from build123d import *

# Parameters (mm, degrees)
SKETCH1_W            = 190.5
SKETCH1_H            = 76.2
BOSS_EXTRUDE1_DEPTH  = 3.175
SKETCH2_R            = 1.545336663
CUT_EXTRUDE4_DEPTH   = 4.175
SKETCH3_W            = 153.75
SKETCH3_H            = 3.175
BOSS_EXTRUDE2_DEPTH  = 3.175
CUT_SWEEP1_PROFILE_R = 12.7


with BuildPart() as part:
    # Sketch1 → Boss-Extrude1 (new body)
    with BuildSketch(Plane(origin=(0, 0, 0), x_dir=(1, 0, 0), z_dir=(0, 1, 0))):
        Rectangle(SKETCH1_W, SKETCH1_H)
    extrude(amount=BOSS_EXTRUDE1_DEPTH)

    # Sketch2 → Cut-Extrude4 (cut, through all)
    with BuildSketch(Plane(origin=(0, 3.175, 0), x_dir=(1, 0, 0), z_dir=(0, 1, 0))):
        Polygon((-58.5, 12.6), (-58.5, -38.1), (95.25, -38.1), (95.25, 38.1), (58.5, 38.1), (58.5, 12.6), (56.5, 12.6), (41.5, 26.6), (41.5, 32.45), (-41.5, 32.45), (-41.5, 26.6), (-56.5, 12.6), align=None)
        with Locations((-52.505245516, 25.605245516)):
            Circle(SKETCH2_R)
        with Locations((52.5, 25.605245516)):
            Circle(SKETCH2_R)
    extrude(amount=-CUT_EXTRUDE4_DEPTH, mode=Mode.SUBTRACT)

    # Sketch3 → Boss-Extrude2 (add)
    with BuildSketch(Plane(origin=(0, 0, -38.1), x_dir=(-1, 0, 0), z_dir=(0, 0, -1))):
        with Locations((18.375, 1.5875)):
            Rectangle(SKETCH3_W, SKETCH3_H)
    extrude(amount=BOSS_EXTRUDE2_DEPTH)

    # Cut-Sweep1: sweep along a curve in space
    with BuildLine() as cut_sweep1_path:
        Line((-96.6, 3.175, 467.883912637), (-96.6, 3.175, -36.654630794))
        Line((-96.6, 3.175, -36.654630794), (-96.6, 3.175, -207.159673584))
    # Cut-Sweep1 profile (on start of the path) → Cut-Sweep1 (sweep, cut)
    with BuildSketch(Plane(origin=(-96.6, 3.175, 467.883912637), x_dir=(0, -1, 0), z_dir=(0, 0, -1))):
        Circle(CUT_SWEEP1_PROFILE_R)
    sweep(path=cut_sweep1_path.line, mode=Mode.SUBTRACT)


solid = part.part
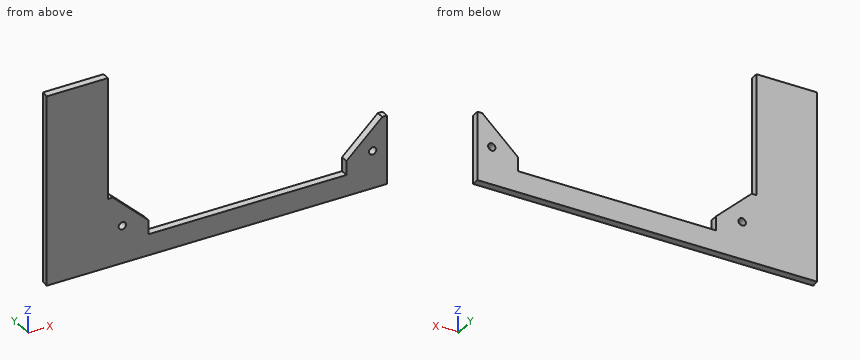
CAD build for the part. Positions are in the model's coordinates, mm. Coordinates: 2 decimals unless noted, no trailing zeros. Order: outer loops, then holes, each group sorted by start corner. A loop starts at its lowest first (then second) coordinate and runs counter-clockwise, first axis right, second up. Notation, with made-up numbers: (-17.75, 35) -> (-13.75, 35) arc R20 cw to (-13.75, 41) -> close; hole circle Ø5 at (-30, 34.5). An arc over 180 degrees is marked (long way). Answer in a Markdown table with one row per item.
1) Band-saw the part on A-A (y = 2.3). List the corners of the cut face in (x, z) (3 decimals), and give its area (3 significant figures).
Check values:
| item | result |
|---|---|
| outline | (-83.93, -41.275) -> (58.5, -41.275) -> (58.5, -12.6) -> (56.5, -12.6) -> (41.5, -26.6) -> (41.5, -32.45) -> (-41.5, -32.45) -> (-41.5, -26.6) -> (-56.5, -12.6) -> (-58.5, -12.6) -> (-58.5, 38.1) -> (-83.93, 38.1) -> close; hole circle Ø3.091 at (-52.505, -25.605); hole circle Ø3.091 at (52.5, -25.605) |
| area | 3,500 mm2 |
2) Drill centre lines: line 1 (Z direction, x = -9, y = 1.95) (3 decimals); line 2 (X direction, y = 2.9, z = -22.5); line 3 (Z direction, x = 52.5, y = 1.4) (3 decimals). Where is each one in solid material? Low to high.
Check values:
| item | result |
|---|---|
| line 1 | -41.275 to -32.45 |
| line 2 | -83.9 to -45.89, 45.89 to 58.5 |
| line 3 | -41.275 to -27.151, -24.06 to -16.333 |
3) Band-saw the part on D-D (z = 20). List the corners of the cut face in (x, y) (3 decimals).
Check values:
| item | result |
|---|---|
| outline | (-84.303, 0) -> (-58.5, 0) -> (-58.5, 3.175) -> (-83.9, 3.175) arc R12.7 cw to start |
4) Band-saw the part on B-B (x = 52.5). List the corners of the cut face in (y, z) (3 decimals).
Check values:
| item | result |
|---|---|
| outline | (0, -41.275) -> (3.175, -41.275) -> (3.175, -27.151) -> (0, -27.151) -> close; (0, -24.06) -> (3.175, -24.06) -> (3.175, -16.333) -> (0, -16.333) -> close |
5) Flat gauge pins, fed straight in: P1, Ø1.6, axis at x = 0, y = 1, coming from the +Z side; P2, Ø1, axis at x = -57, y = 1, coming from the +Z side; P3, Ø3, axis at x = -52.51, z = -25.61, coming from the +Y side; P4, Ø1.5, axis at y = 3, z = 8, coming from the -X side. Where does each tip first touch, or does it go through?
Check values:
| item | result |
|---|---|
| P1 | z = -32.45 |
| P2 | z = -12.6 |
| P3 | through |
| P4 | x = -83.93 |
6) Band-saw the part on C-C (x = 9). List the corners of the cut face in (y, z) (3 decimals).
Check values:
| item | result |
|---|---|
| outline | (0, -41.275) -> (3.175, -41.275) -> (3.175, -32.45) -> (0, -32.45) -> close |
